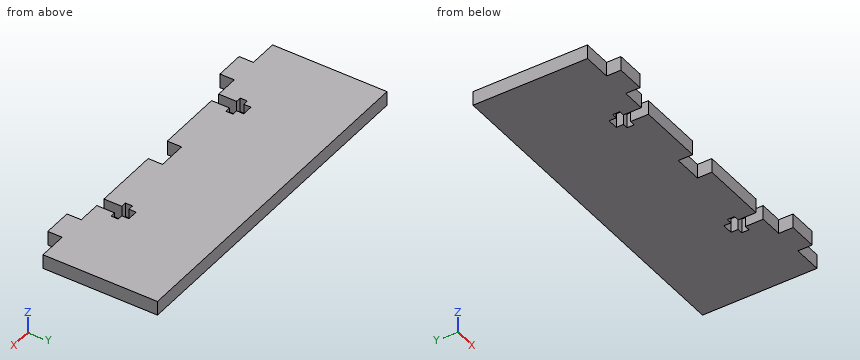
```python
from build123d import *

# Parameters (mm, degrees)
BOSS_EXTRUDE1_DEPTH = 6.35
SKETCH2_W           = 12.7
SKETCH2_H           = 6.35
CUT_EXTRUDE1_DEPTH  = 6.35


with BuildPart() as part:
    # Sketch1 → Boss-Extrude1 (new body)
    with BuildSketch(Plane.XY):
        Polygon((139.7, 6.35), (152.4, 6.35), (152.4, 57.15), (0, 57.15), (0, 6.35), (12.7, 6.35), (12.7, 0), (25.4, 0), (25.4, 6.35), (127, 6.35), (127, 0), (139.7, 0), align=None)
    extrude(amount=BOSS_EXTRUDE1_DEPTH)

    # Sketch2 → Cut-Extrude1 (cut)
    with BuildSketch(Plane.XY.offset(6.35)):
        Polygon((111.91875, 6.35), (111.91875, 14.2875), (109.5375, 14.2875), (109.5375, 17.4625), (111.91875, 17.4625), (111.91875, 20.6375), (116.68125, 20.6375), (116.68125, 17.4625), (119.0625, 17.4625), (119.0625, 14.2875), (116.68125, 14.2875), (116.68125, 6.35), align=None)
        Polygon((42.8625, 17.4625), (42.8625, 14.2875), (40.48125, 14.2875), (40.48125, 6.35), (35.71875, 6.35), (35.71875, 14.2875), (33.3375, 14.2875), (33.3375, 17.4625), (35.71875, 17.4625), (35.71875, 20.6375), (40.48125, 20.6375), (40.48125, 17.4625), align=None)
        with Locations((76.2, 9.525)):
            Rectangle(SKETCH2_W, SKETCH2_H)
    extrude(amount=-CUT_EXTRUDE1_DEPTH, mode=Mode.SUBTRACT)


solid = part.part
```
Work out the finished part from the listing and answer in its coordinate system (mm). Give positions to 0.01 mm unless a question says otherwise; leave off trailing zeros. Loops run counter-clockwise (first coordinate to the right, second up) from the corner with the lowest first, then second, coordinate; pieces in that order, holes last. Notation, with made-up numbers: (30, 37.5) - (39, 37.5) arc R23 ccw to (39, 58.5) - close; hole circle Ø7 at (7, 82.25). An arc over 180 degrees is marked (long way). One line per question, with ' | ' between items.
(1) The part is cut by section A-A (y = 8.5). Write down the section's boundary in (x, z), then the cut area to 3 significant figures.
Recorded:
outline: (0, 0) - (35.72, 0) - (35.72, 6.35) - (0, 6.35) - close; (40.48, 0) - (69.85, 0) - (69.85, 6.35) - (40.48, 6.35) - close; (82.55, 0) - (111.92, 0) - (111.92, 6.35) - (82.55, 6.35) - close; (116.68, 0) - (152.4, 0) - (152.4, 6.35) - (116.68, 6.35) - close | area: 827 mm²
(2) The part is cut by section C-C (x = 81). Write down the section's boundary in (y, z).
Recorded:
outline: (12.7, 0) - (57.15, 0) - (57.15, 6.35) - (12.7, 6.35) - close
(3) Each of these flat-tipped pins is pushed along its axis until it touches: pin 1 Ø1.9 at (x, z) = (118.5, 4) entering from -Y; pin 2 Ø1.9 at (y, z) = (3.5, 4) entering from +X; pin 3 Ø3 at (x, z) = (70, 1) entering from -Y. Where does it stop, or does it pass through?
Recorded:
pin 1: stops at y = 6.35 | pin 2: stops at x = 139.7 | pin 3: stops at y = 6.35
(4) Straight lines are drawn through the part: probe 1 along X at (y, z) = (12.5, 3); probe 2 along X at (y, z) = (13, 1.75); probe 3 along X at (y, z) = (4.5, 2.25). For each, find the intervals that lie inside material, in ascending order.
Recorded:
probe 1: x = 0 to 35.72, 40.48 to 69.85, 82.55 to 111.92, 116.68 to 152.4 | probe 2: x = 0 to 35.72, 40.48 to 111.92, 116.68 to 152.4 | probe 3: x = 12.7 to 25.4, 127 to 139.7
(5) The part is cut by section B-B (x = 107). Write down the section's boundary in (y, z).
Recorded:
outline: (6.35, 0) - (57.15, 0) - (57.15, 6.35) - (6.35, 6.35) - close
